```python
from build123d import *

# Parameters (mm, degrees)
EXTRUDE_1_DEPTH     = 5
EXTRUDE_2_DEPTH     = 35
SKETCH_4_W          = 116
SKETCH_4_H          = 31.7
EXTRUDE_3_DEPTH     = 3
SKETCH_6_R          = 5
CUT_EXTRUDE_1_DEPTH = 190.221017262


with BuildPart() as part:
    # 草图2 → 凸台-拉伸1 (new body)
    with BuildSketch(Plane.XY):
        Polygon((-30.006166306, -35.96646266), (29.993833694, -35.96646266), (29.993833694, -144.35646266), (57.993833694, -144.35646266), (57.993833694, -176.05646266), (-58.006166306, -176.05646266), (-58.006166306, -144.35646266), (-30.006166306, -144.35646266), align=None)
    extrude(amount=EXTRUDE_1_DEPTH)

    # 草图3 → 凸台-拉伸2 (add)
    with BuildSketch(Plane(origin=(0, 0, 0), x_dir=(-1, 0, 0), z_dir=(0, 0, -1))):
        Polygon((-57.993833694, -144.35646266), (-57.993833694, -176.05646266), (58.006166306, -176.05646266), (58.006166306, -144.35646266), (55.006166306, -144.35646266), (55.006166306, -173.05646266), (-54.993833694, -173.05646266), (-54.993833694, -144.35646266), align=None)
    extrude(amount=EXTRUDE_2_DEPTH)

    # 草图4 → 凸台-拉伸3 (add)
    with BuildSketch(Plane(origin=(0, 0, -35), x_dir=(-1, 0, 0), z_dir=(0, 0, -1))):
        with Locations((0.006166306, -160.20646266)):
            Rectangle(SKETCH_4_W, SKETCH_4_H)
    extrude(amount=EXTRUDE_3_DEPTH)

    # 草图6 → 切除-拉伸1 (cut, through all)
    with BuildSketch(Plane(origin=(0, 0, 0), x_dir=(-1, 0, 0), z_dir=(0, 0, -1))):
        with Locations((-17.993833694, -47.96646266)):
            Circle(SKETCH_6_R)
        with Locations(Location((18.006166306, -47.96646266, 0), (0, 0, 180))):
            Circle(SKETCH_6_R)
    extrude(amount=-CUT_EXTRUDE_1_DEPTH, mode=Mode.SUBTRACT)


solid = part.part
```
Here's how the part is built. I have some questions about the finished solid (model axes, mm). A direction names the side the tool comes from. Give positions to 0.01 mm unless a question says otherwise; leave off trailing zeros. Order: outer loops, then holes, each group sorted by start corner. A loop starts at its lowest first (then second) coordinate and runs counter-clockwise, first axis right, second up. Notation, with made-up numbers: M -31.5,15.5 L 17.5,15.5 A12 cw 17.5,25.5 Z; hole C -36.5,60.5 d2. An arc over 180 degrees is marked long. Use a Markdown table: item, result. Add a question column.
1. Suppose I cut it at A-A (x = -16). List the corners of the cut face in (y, z) for me.
2. Suppose I cut it at C-C (z = -30). List the corners of the cut face in (x, y) for me, and give its area (3 significant figures).
3. Suppose I cut it at D-D (x = 11). List the corners of the cut face in (y, z) for me, and give its area (3 significant figures).
4. Suppose I cut it at B-B (y = -157). List the corners of the cut face in (x, z) for me.
5. For pin 1 Ø13 at (x, y) = (17.99, -47.97) entering from +Z; pin 2 Ø1 at (x, y) = (12.5, -76) entering from -Z; pin 3 Ø4 at (y, z) = (-86.5, 3.5) entering from -X; pin 4 Ø4 at (y, z) = (-97, 1.5) entering from +X, each with a flat end and sliding along its axis, tell me the tip position at first contact or that it passes through.
6. I need wall thicknesses on probe 1 along X at (y, z) = (-157, -33); probe 2 along Z at (x, y) = (-51, -168.5); probe 3 along Y at (x, z) = (27, -7). Which ranges of each line are inside material? Lowest first, please. Write a range as from..to.
7. If we mould it in two halves opening along Y, with no side actions, what happens to faces 1 (the cylindrical face through (-21.69, -51.35, 2.46)), 2 (the flat face through (1, -119, 0)), 3 (the flat face through (1, -176.056, -16))? For each: +Y half, -Y half, draft (parallel to the pull), parting line (faces both ways), or undercut.
8. On a 3-axis mill with a long thin cutter (end or side, diameter ignored), from which of +Z, -Z, +X, -X, +Y, -Y can I reach the whole of each face in a straight line? I mean faces 4 (the flat face through (-1, -173.056, -17)), 5 (the flat face through (0, -144.356, -36)), 6 (the flat face through (-30.006, -91, 2)), 7 (the flat face through (29.994, -89, 2)). Say none if no direction works.
Results list:
| question | item | result |
|---|---|---|
| 1 | outline | M -176.06,-38 L -144.36,-38 L -144.36,-35 L -173.06,-35 L -173.06,0 L -52.55,0 L -52.55,5 L -176.06,5 Z; M -43.39,0 L -35.97,0 L -35.97,5 L -43.39,5 Z |
| 2 | outline | M -58.01,-176.06 L 57.99,-176.06 L 57.99,-144.36 L 54.99,-144.36 L 54.99,-173.06 L -55.01,-173.06 L -55.01,-144.36 L -58.01,-144.36 Z |
| 2 | area | 520 mm² |
| 3 | outline | M -176.06,-38 L -144.36,-38 L -144.36,-35 L -173.06,-35 L -173.06,0 L -35.97,0 L -35.97,5 L -176.06,5 Z |
| 3 | area | 901 mm² |
| 4 | outline | M -58.01,-38 L 57.99,-38 L 57.99,5 L -58.01,5 Z; hole M -55.01,-35 L 54.99,-35 L 54.99,0 L -55.01,0 Z |
| 5 | pin 1 | stops at z = 5 |
| 5 | pin 2 | stops at z = 0 |
| 5 | pin 3 | stops at x = -30.01 |
| 5 | pin 4 | stops at x = 29.99 |
| 6 | probe 1 | x = -58.01..-55.01, 54.99..57.99 |
| 6 | probe 2 | z = -38..-35, 0..5 |
| 6 | probe 3 | y = -176.06..-173.06 |
| 7 | face 1 | undercut |
| 7 | face 2 | draft |
| 7 | face 3 | -Y half |
| 8 | face 4 | +Y |
| 8 | face 5 | -Z, +Y |
| 8 | face 6 | +Z, -Z, -X, +Y |
| 8 | face 7 | +Z, -Z, +X, +Y |
